Verification items for the finished model (mm, model axes). Face numbers are marked on the shaded views. A direction names the side the tool comes from. Give positions to 0.01 mm unless a question says otherwise; leave off trailing zeros. Order: outer loops, then holes, each group sorted by start corner. A loop starts at its lowest first (then second) coordinate and runs counter-clockwise, first axis right, second up. Notation, with made-up numbers: (68.25, -10.5) - (108.25, -10.5) arc R20 ccw to (108.25, 0.5) - close; hole circle Ø6 at (36, 54.25). An arc over 180 degrees is marked (long way). Answer as a JSON object with one key per item and string values.
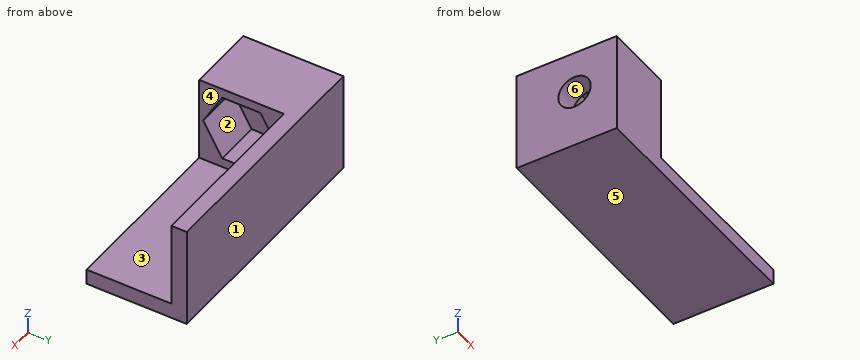
```python
from build123d import *

# Parameters (mm, degrees)
SKETCH_1_W          = 32
SKETCH_1_H          = 13
EXTRUDE_1_DEPTH     = 2
SKETCH_2_W          = 32
SKETCH_2_H          = 2
EXTRUDE_2_DEPTH     = 11
SKETCH_3_W          = 9
SKETCH_3_H          = 11
EXTRUDE_3_DEPTH     = 11
CUT_EXTRUDE_1_DEPTH = 6
SKETCH_5_R          = 2.1
CUT_EXTRUDE_2_DEPTH = 3


with BuildPart() as part:
    # 草图1 → 凸台-拉伸1 (new body)
    with BuildSketch(Plane(origin=(0, 0, 0), x_dir=(1, 0, 0), z_dir=(0, 1, 0))):
        with Locations((2.487093154, 5.054433221)):
            Rectangle(SKETCH_1_W, SKETCH_1_H)
    extrude(amount=EXTRUDE_1_DEPTH)

    # 草图2 → 凸台-拉伸2 (add)
    with BuildSketch(Plane(origin=(0, 0, 0), x_dir=(-1, 0, 0), z_dir=(0, -1, 0))):
        with Locations((-2.487093154, 10.554433221)):
            Rectangle(SKETCH_2_W, SKETCH_2_H)
    extrude(amount=EXTRUDE_2_DEPTH)

    # 草图3 → 凸台-拉伸3 (add)
    with BuildSketch(Plane.XZ):
        with Locations((-9.012906846, -4.054433221)):
            Rectangle(SKETCH_3_W, SKETCH_3_H)
    extrude(amount=EXTRUDE_3_DEPTH)

    # 草图4 → 切除-拉伸1 (cut)
    with BuildSketch(Plane(origin=(-4.512906846, 0, 0), x_dir=(0, 0, -1), z_dir=(1, 0, 0))):
        Polygon((4.054433221, -10.48042463), (8.354433221, -7.997818473), (8.354433221, -3.032606158), (4.054433221, -0.55), (-0.245566779, -3.032606158), (-0.245566779, -7.997818473), align=None)
    extrude(amount=-CUT_EXTRUDE_1_DEPTH, mode=Mode.SUBTRACT)

    # 草图5 → 切除-拉伸2 (cut)
    with BuildSketch(Plane(origin=(-10.512906846, 0, 0), x_dir=(0, 0, -1), z_dir=(1, 0, 0))):
        with Locations((4.054433221, -5.515212315)):
            Circle(SKETCH_5_R)
    extrude(amount=-CUT_EXTRUDE_2_DEPTH, mode=Mode.SUBTRACT)


solid = part.part
```
(1) Gauge pin test, flat ends, axial feed: pin 1 Ø3 at (x, z) = (12, -5.5) entering from -Y; pin 2 Ø5.5 at (y, z) = (-7.5, -2) entering from +X. Record the tip position at first contact, or that the pin passes through.
Computed values:
{"pin 1": "stops at y = 0", "pin 2": "stops at x = -4.51"}
(2) Access from +Z, -Z, +X, -X, +Y, -Y to the whole of each face (thin tool, end or side, straight path). Record for the marked faces 1, 2 and 3.
Computed values:
{"face 1": "+Z, -Z, +X, -X, +Y", "face 2": "+X", "face 3": "+Z, +X, -Y"}
(3) Section check B-B (z = -5.75). Record the cut outline in (x, y), then the cut area to 3 significant figures.
Computed values:
{"outline": "(-13.51, -11) - (-4.51, -11) - (-4.51, -9.5) - (-10.51, -9.5) - (-10.51, -6.75) - (-13.51, -6.75) - close; (-13.51, -4.28) - (-10.51, -4.28) - (-10.51, -1.53) - (-4.51, -1.53) - (-4.51, 0) - (18.49, 0) - (18.49, 2) - (-13.51, 2) - close", "area": "108 mm²"}
(4) Section check C-C (y = -7.25). Record the cut outline in (x, z), then the cut area to 3 significant figures.
Computed values:
{"outline": "(-13.51, -11.55) - (18.49, -11.55) - (18.49, -9.55) - (-4.51, -9.55) - (-4.51, -8.35) - (-10.51, -8.35) - (-10.51, -5.24) - (-13.51, -5.24) - close; (-13.51, -2.87) - (-10.51, -2.87) - (-10.51, 0.25) - (-4.51, 0.25) - (-4.51, 1.45) - (-13.51, 1.45) - close", "area": "104 mm²"}
(5) Material ranges on line 1 along Z through (x, y) = (-9, -5.75); line 2 along Y through (x, z) = (2, -7); line 3 along Z through (x, y) = (-4, -5), recorded low to high. Write a range as [from, to].
Computed values:
{"line 1": "z = [-11.55, -8.35], [0.25, 1.45]", "line 2": "y = [0, 2]", "line 3": "z = [-11.55, -9.55]"}
(6) Section check A-A (x = -7). Record the cut outline in (y, z), then the cut area to 3 significant figures.
Computed values:
{"outline": "(-11, -11.55) - (2, -11.55) - (2, 1.45) - (-11, 1.45) - close; hole (-10.48, -4.05) - (-8, -8.35) - (-3.03, -8.35) - (-0.55, -4.05) - (-3.03, 0.25) - (-8, 0.25) - close", "area": "105 mm²"}
(7) Release check for a two-part mould opening along Z. For the marked faces 4, 5 and 6 record: pulls with the +Z half, pulls with the -Z half, needs draft (parallel to the pull), parting line crosses it, or undercut.
Computed values:
{"face 4": "needs draft", "face 5": "pulls with the -Z half", "face 6": "undercut"}
(8) Section check D-D (x = 6.5). Record the cut outline in (y, z).
Computed values:
{"outline": "(-11, -11.55) - (2, -11.55) - (2, 1.45) - (0, 1.45) - (0, -9.55) - (-11, -9.55) - close"}
